Geometry: final body of the model. Coordinates: model frame, mm. Face numbers are marked on the shaded views. A direction names the side the tool comes from. Give positions to 0.01 mm unless a question says otherwise; leave off trailing zeros. Order: outer loops, then holes, each group sorted by start corner. A loop starts at its lowest first (then second) coordinate and runs counter-clockwise, first axis right, second up. Notation, with made-up numbers: (60, 24) -> (65, 24) arc R19 ccw to (65, 45) -> close; hole circle Ø1 at (63.5, 42.25). An arc over 180 degrees is marked (long way). Answer in a Markdown table with one row per item. Add a question column.
Q1. Cut plane C-C on z = 12.25. Return the cut outline in (x, y).
Q2. Contact query for flat-ended pins moving along their axis: P1, Ø1.5, axis at y = -3.5, z = -6.5, coming from the +X side; P2, Ø7, axis at x = 0, z = 0, coming from the +Y side; P3, Ø3.5, axis at x = 0, y = 1, coming from the +Z side. Output: stop coordinate, or through.
Q3. Line query: line 1 along X through (y, z) = (5, 0); line 2 along Y through (x, z) = (5.75, -12); line 3 along Z through (x, y) = (0, 3.5). Output: solid intervals per line, ascending. Write a range as from..to.
Q4. Cut plane A-A on x = 0. Return the cut outline in (y, z), and give its area (3 significant figures).
Q5. Cut plane D-D on z = 3.25. Return the cut outline in (x, y), and give its area (3 significant figures).
Q6. Cut plane B-B on y = 1. Return the cut outline in (x, z).
Q7. Pull-direction query (Y, two-part tool) for the marked faces 3, 4 and 5; classes: +Y half, -Y half, draft (parallel to the pull), parting line (faces both ways), or undercut.
Q8. Set-up query: the marked faces 1 and 2. Return all of +Z, -Z, +X, -X, +Y, -Y with unobstructed straight access to the full face (end or side cutting, diameter ignored); none if empty.
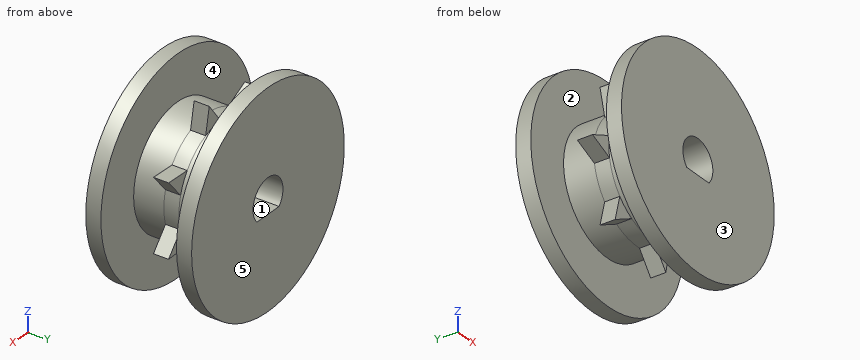
Autodesk Inventor part; units mm, degrees
ref_plane "YZ Plane" through (0, 0, 0) normal (1, 0, 0) x (0, 1, 0)
ref_plane "XZ Plane" through (0, 0, 0) normal (0, 1, 0) x (-1, 0, 0)
ref_plane "XY Plane" through (0, 0, 0) normal (0, 0, 1) x (1, 0, 0)
sketch "Sketch1" plane through (0, 0, 0) normal (0, 1, 0) x (-1, 0, 0)
  line L0 (0, 0) -> (13.4559, 0) construction
  line L1 (7.8785, 1.3892) -> (11, 0)
  line L2 (7.8785, -1.3892) -> (11, 0)
  line L3 (5.9982, 5.2935) -> (6.8584, 8.6001)
  line L4 (3.826, 7.0258) -> (6.8584, 8.6001)
  line L5 (-0.3988, 7.9901) -> (-2.4477, 10.7242)
  line L6 (-3.1075, 7.3718) -> (-2.4477, 10.7242)
  line L7 (-6.4955, 4.6699) -> (-9.9107, 4.7727)
  line L8 (-7.701, 2.1667) -> (-9.9107, 4.7727)
  line L9 (-7.701, -2.1667) -> (-9.9107, -4.7727)
  line L10 (-6.4955, -4.6699) -> (-9.9107, -4.7727)
  line L11 (-3.1075, -7.3718) -> (-2.4477, -10.7242)
  line L12 (-0.3988, -7.9901) -> (-2.4477, -10.7242)
  line L13 (3.826, -7.0258) -> (6.8584, -8.6001)
  line L14 (5.9982, -5.2935) -> (6.8584, -8.6001)
  arc A0 (7.8785, 1.3892) -> (5.9982, 5.2935) centre (0, 0) ccw
  arc A1 (5.9982, -5.2935) -> (7.8785, -1.3892) centre (0, 0) ccw
  arc A2 (-0.3988, -7.9901) -> (3.826, -7.0258) centre (0, 0) ccw
  arc A3 (-6.4955, -4.6699) -> (-3.1075, -7.3718) centre (0, 0) ccw
  arc A4 (-7.701, 2.1667) -> (-7.701, -2.1667) centre (0, 0) ccw
  arc A5 (3.826, 7.0258) -> (-0.3988, 7.9901) centre (0, 0) ccw
  arc A6 (-3.1075, 7.3718) -> (-6.4955, 4.6699) centre (0, 0) ccw
  dimension "d10" = 360
extrude "Extrusion1" add sketch "Sketch1" along normal blind 2
sketch "Sketch2" plane through (0, 2, 0) normal (0, 1, 0) x (1, 0, 0)
  circle A0 centre (0, 0) radius 8
extrude "Extrusion2" add sketch "Sketch2" along normal blind 4
sketch "Sketch3" plane through (0, 0, 0) normal (0, -1, 0) x (1, 0, 0)
  circle A0 centre (0, 0) radius 8
extrude "Extrusion3" add sketch "Sketch3" along normal blind 4
sketch "Sketch4" plane through (0, 6, 0) normal (0, 1, 0) x (1, 0, 0)
  circle A0 centre (0, 0) radius 14
  dimension "d18" = 28
sketch "Sketch5" plane through (0, -4, 0) normal (0, -1, 0) x (1, 0, 0)
  circle A0 centre (0, 0) radius 14
  dimension "d19" = 28
extrude "Extrusion4" add sketch "Sketch5" along normal blind 2
extrude "Extrusion5" add sketch "Sketch4" along normal blind 2
sketch "Sketch6" plane through (0, 8, 0) normal (0, 1, 0) x (1, 0, 0)
  arc A0 (-2.0347, 1.85) -> (2.0347, 1.85) centre (0, 0) ccw
  line L0 (-2.0347, 1.85) -> (2.0347, 1.85)
  dimension "d24" = 5.5
extrude "Extrusion6" cut sketch "Sketch6" against normal through all
Completed:
| question | item | result |
|---|---|---|
| 1 | outline | (-6.78, -6) -> (6.78, -6) -> (6.78, -4) -> (-6.78, -4) -> close; (-6.78, 6) -> (6.78, 6) -> (6.78, 8) -> (-6.78, 8) -> close |
| 2 | P1 | stops at x = 12.68 |
| 2 | P2 | stops at y = 8 |
| 2 | P3 | stops at z = 9.79 |
| 3 | line 1 | x = -8..-2.75, 2.75..8 |
| 3 | line 2 | y = -6..-4, 6..8 |
| 3 | line 3 | z = -8..-1.85, 2.75..8 |
| 4 | outline | (-6, -14) -> (-4, -14) -> (-4, -8) -> (0, -8) -> (6, -8) -> (6, -14) -> (8, -14) -> (8, -1.85) -> (-6, -1.85) -> close; (-6, 2.75) -> (8, 2.75) -> (8, 14) -> (6, 14) -> (6, 8) -> (0, 8) -> (-4, 8) -> (-4, 14) -> (-6, 14) -> close |
| 4 | area | 208 mm² |
| 5 | outline | (-13.62, -6) -> (13.62, -6) -> (13.62, -4) -> (7.31, -4) -> (7.31, 0) -> (8.62, 0) -> (8.62, 2) -> (7.31, 2) -> (7.31, 6) -> (13.62, 6) -> (13.62, 8) -> (-13.62, 8) -> (-13.62, 6) -> (-7.31, 6) -> (-7.31, 0) -> (-7.31, -4) -> (-13.62, -4) -> close |
| 5 | area | 258 mm² |
| 6 | outline | (-11, 0) -> (-7.88, -1.39) arc R8 ccw to (-6, -5.29) -> (-6.86, -8.6) -> (-3.83, -7.03) arc R8 ccw to (0.4, -7.99) -> (2.45, -10.72) -> (3.11, -7.37) arc R8 ccw to (6.5, -4.67) -> (9.91, -4.77) -> (7.7, -2.17) arc R8 ccw to (7.7, 2.17) -> (9.91, 4.77) -> (6.5, 4.67) arc R8 ccw to (3.11, 7.37) -> (2.45, 10.72) -> (0.4, 7.99) arc R8 ccw to (-3.83, 7.03) -> (-6.86, 8.6) -> (-6, 5.29) arc R8 ccw to (-7.88, 1.39) -> close; hole (-2.03, -1.85) -> (2.03, -1.85) arc R2.75 ccw (long way) to start |
| 7 | face 3 | -Y half |
| 7 | face 4 | undercut |
| 7 | face 5 | +Y half |
| 8 | face 1 | +Y, -Y |
| 8 | face 2 | none |
